CAD build for the part. Positions are in the model's coordinates, mm. A direction names the side the tool comes from. Round coordinates to 2 decimals unless told otherwise and drop trailing zeros. Loops run counter-clockwise (first coordinate to the right, second up) from the corner with the lowest first, then second, coordinate; pieces in that order, holes last.
from build123d import *

# Parameters (mm, degrees)
F1_DEPTH    = 3.175
F2_T1_DEPTH = 41.9033921872
F3_T1_DEPTH = 42.5180012054
F4_T1_DEPTH = 41.9033921872
F5_T1_DEPTH = 41.9033921872


# Not quite as in the source:
# - a fillet or chamfer that OpenCascade refuses, or shapes differently, is made with other operations: its cross-section is extruded or revolved along the edge and cut away or added
# - ends of sketch curves that miss each other by under 0.0002 mm in the source are joined


with BuildPart() as f1:
    # F0 (on Front) → F1 (new body)
    with BuildSketch(Plane.XZ):
        Polygon((-134.9552678654, 118.4551059571), (-242.3083075974, 118.4551059571), (-264.8317917845, 79.4432945156), (-264.8317917845, 5.0669305831), (-242.3083075974, -33.9448883924), (-264.8317917845, -72.9567073679), (-264.8317917845, -147.3330713004), (-242.3083075974, -186.3448902759), (-264.8317917845, -225.3567092514), (-264.8317917845, -299.7330731839), (-242.3083075974, -338.7448921594), (-264.8317917845, -377.7567111349), (-264.8317917845, -452.1330750674), (-242.3083075974, -491.1448940429), (-134.9552678654, -491.1448940429), (-98.2935257718, -427.6448940429), (-24.9700415847, -427.6448940429), (11.6917005088, -491.1448940429), (119.0447402409, -491.1448940429), (155.7064823344, -427.6448940429), (192.3682082155, -427.6448940429), (192.3682082155, -402.2448921594), (155.7064823344, -402.2448921594), (119.0447402409, -338.7448921594), (155.7064823344, -275.2448921594), (192.3682082155, -275.2448921594), (192.3682082155, -249.8448902759), (155.7064823344, -249.8448902759), (119.0447402409, -186.3448902759), (155.7064823344, -122.8448902759), (192.3682082155, -122.8448902759), (192.3682082155, -97.4448883924), (155.7064823344, -97.4448883924), (119.0447402409, -33.9448883924), (155.7064823344, 29.5551116076), (192.3682082155, 29.5551116076), (192.3682082155, 54.9551134911), (155.7064823344, 54.9551134911), (119.0447402409, 118.4551134911), (11.6917005088, 118.4551059571), (-24.9700415847, 54.9551134911), (-98.2935257718, 54.9551134911), align=None)
        Polygon((-261.9552759716, -414.9448940429), (-225.2935338781, -351.4448940429), (-151.970049691, -351.4448940429), (-115.3083075974, -414.9448940429), (-151.970049691, -478.4448940429), (-225.2935338781, -478.4448940429), align=None, mode=Mode.SUBTRACT)
        Polygon((11.6917005088, -338.7448921594), (-24.9700415847, -402.2448921594), (-98.2935257718, -402.2448921594), (-134.9552678654, -338.7448921594), (-98.2935257718, -275.2448921594), (-24.9700415847, -275.2448921594), align=None, mode=Mode.SUBTRACT)
        Polygon((-115.3083075974, -262.5448921594), (-151.970049691, -326.0448921594), (-225.2935338781, -326.0448921594), (-261.9552759716, -262.5448921594), (-225.2935338781, -199.0448921594), (-151.970049691, -199.0448921594), align=None, mode=Mode.SUBTRACT)
        Polygon((138.6917005088, -414.9448940429), (102.0299584153, -478.4448940429), (28.7064742282, -478.4448940429), (-7.9552678654, -414.9448940429), (28.7064742282, -351.4448940429), (102.0299584153, -351.4448940429), align=None, mode=Mode.SUBTRACT)
        Polygon((138.6917005088, -262.5448921594), (102.0299584153, -326.0448921594), (28.7064742282, -326.0448921594), (-7.9552678654, -262.5448921594), (28.7064742282, -199.0448921594), (102.0299584153, -199.0448921594), align=None, mode=Mode.SUBTRACT)
        Polygon((-115.3083075974, -110.1448902759), (-151.970049691, -173.6448902759), (-225.2935338781, -173.6448902759), (-261.9552759716, -110.1448902759), (-225.2935338781, -46.6448902759), (-151.970049691, -46.6448902759), align=None, mode=Mode.SUBTRACT)
        Polygon((11.6917005088, -186.3448902759), (-24.9700415847, -249.8448902759), (-98.2935257718, -249.8448902759), (-134.9552678654, -186.3448902759), (-98.2935257718, -122.8448902759), (-24.9700415847, -122.8448902759), align=None, mode=Mode.SUBTRACT)
        Polygon((11.6917005088, -33.9448883924), (-24.9700415847, -97.4448883924), (-98.2935257718, -97.4448883924), (-134.9552678654, -33.9448883924), (-98.2935257718, 29.5551116076), (-24.9700415847, 29.5551116076), align=None, mode=Mode.SUBTRACT)
        Polygon((-115.3083075974, 42.2551116076), (-151.970049691, -21.2448883924), (-225.2935338781, -21.2448883924), (-261.9552759716, 42.2551116076), (-225.2935338781, 105.7551116076), (-151.970049691, 105.7551116076), align=None, mode=Mode.SUBTRACT)
        Polygon((138.6917005088, -110.1448902759), (102.0299584153, -173.6448902759), (28.7064742282, -173.6448902759), (-7.9552678654, -110.1448902759), (28.7064742282, -46.6448902759), (102.0299584153, -46.6448902759), align=None, mode=Mode.SUBTRACT)
        Polygon((138.6917005088, 42.2551116076), (102.0299584153, -21.2448883924), (28.7064742282, -21.2448883924), (-7.9552678654, 42.2551116076), (28.7064742282, 105.7551116076), (102.0299584153, 105.7551116076), align=None, mode=Mode.SUBTRACT)
    extrude(amount=F1_DEPTH)

    # F2: chamfer of 1.8415 x 3.1895715621 on 1 edges, made by hand

    # F2_s2 → F2_t1 (cut)
    with BuildSketch(Plane.XY.offset(21.3034164558)):
        Polygon((192.3682082155, -3.1895715621), (190.5267082155, 0), (192.3682082155, 0), align=None)
    extrude(amount=F2_T1_DEPTH, mode=Mode.SUBTRACT)

    # F3: chamfer of 1.91008 x 3.3083556065 on 1 edges, made by hand

    # F3_s2 → F3_t1 (cut)
    with BuildSketch(Plane.XY.offset(-131.4038899368)):
        Polygon((190.4581282155, 0), (192.3682082155, -3.3083556065), (192.3682082155, 0), align=None)
    extrude(amount=F3_T1_DEPTH, mode=Mode.SUBTRACT)

    # F4: chamfer of 1.8415 x 3.1895715621 on 1 edges, made by hand

    # F4_s2 → F4_t1 (cut)
    with BuildSketch(Plane.XY.offset(-283.4965873112)):
        Polygon((190.5267082155, 0), (192.3682082155, -3.1895715621), (192.3682082155, 0), align=None)
    extrude(amount=F4_T1_DEPTH, mode=Mode.SUBTRACT)

    # F5: chamfer of 1.8415 x 3.1895715621 on 1 edges, made by hand

    # F5_s2 → F5_t1 (cut)
    with BuildSketch(Plane.XY.offset(-435.8965891948)):
        Polygon((190.5267082155, 0), (192.3682082155, -3.1895715621), (192.3682082155, 0), align=None)
    extrude(amount=F5_T1_DEPTH, mode=Mode.SUBTRACT)


solid = f1.part
Item 1: Mould opens along X. For faces 1 (the flat face through (-253.728, -1.565, -14.166)), 2 (the flat face through (137.12, -1.57, -459.84)), 3 (the flat face through (120.617, -1.565, 10.95)) say: released by +X, released by -X, zero draft, split by the parting line, or undercut.
Verdict:
face 1: released by -X
face 2: released by +X
face 3: undercut
Item 2: Wall check: L1, parallel to Z at x = -37.5, y = -1.55; L2, parallel to Z at x = -163, y = -1.45; L3, parallel to X at y = -2.25, z = -119.5. Give the ranges that are in metal, low to high.
Verdict:
L1: z = -427.64 to -402.24, -275.24 to -249.84, -122.84 to -97.44, 29.56 to 54.96
L2: z = -491.14 to -478.44, -351.44 to -326.04, -199.04 to -173.64, -46.64 to -21.24, 105.76 to 118.46
L3: x = -264.83 to -256.55, -120.71 to -2.55, 133.29 to 191.76
Item 3: Cut at D-D (x = -176). List the corners of the cut face in (y, z) (3 decimals).
Verdict:
outline: (-3.175, -491.145) - (0, -491.145) - (0, -478.445) - (-3.175, -478.445) - close; (-3.175, -351.445) - (0, -351.445) - (0, -326.045) - (-3.175, -326.045) - close; (-3.175, -199.045) - (0, -199.045) - (0, -173.645) - (-3.175, -173.645) - close; (-3.175, -46.645) - (0, -46.645) - (0, -21.245) - (-3.175, -21.245) - close; (-3.175, 105.755) - (0, 105.755) - (0, 118.455) - (-3.175, 118.455) - close
Item 4: Flat gauge pins, fed straight in: P1, Ø1, axis at x = -79.5, y = -1, coming from the +Z side; P2, Ø1.6, axis at x = -78, y = -1, coming from the -Z side. Where does each tip first touch, or does it go through?
Verdict:
P1: stops at z = 54.96
P2: stops at z = -427.64
Item 5: Cut at B-B (z = -281.5). List the corners of the cut face in (x, y) (3 decimals), plus the area to 3 significant figures.
Verdict:
outline: (-264.832, -3.175) - (-251.012, -3.175) - (-251.012, 0) - (-264.832, 0) - close; (-126.252, -3.175) - (-101.905, -3.175) - (-101.905, 0) - (-126.252, 0) - close; (-21.359, -3.175) - (2.988, -3.175) - (2.988, 0) - (-21.359, 0) - close; (127.748, -3.175) - (152.095, -3.175) - (152.095, 0) - (127.748, 0) - close
area: 276 mm2
Item 6: Cut at C-C (x = 129.5). State how many separate pieces and enclosed holes the cut face has, plus the area to 3 significant figures.
Verdict:
separate pieces: 8
enclosed holes: 0
area: 1,070 mm2
Item 7: 3-axis set-ups, long thin cutter, end or side, ignore diameter. For faces 4 (the flat face through (-6.383, -1.565, 87.15)), 5 (the flat face through (137.12, -1.57, -2.64)), 6 (the flat face through (10.632, -1.565, 10.061)): which of +Z, -Z, +X, -X, +Y, -Y reach the whole face in a straight line?
Verdict:
face 4: +Z, +Y, -Y
face 5: +X, +Y, -Y
face 6: +Y, -Y
Item 8: Cut at A-A (x = -66.5). List the corners of the cut face in (y, z) (3 decimals), plus the area to 3 significant figures.
Verdict:
outline: (-3.175, -427.645) - (0, -427.645) - (0, -402.245) - (-3.175, -402.245) - close; (-3.175, -275.245) - (0, -275.245) - (0, -249.845) - (-3.175, -249.845) - close; (-3.175, -122.845) - (0, -122.845) - (0, -97.445) - (-3.175, -97.445) - close; (-3.175, 29.555) - (0, 29.555) - (0, 54.955) - (-3.175, 54.955) - close
area: 323 mm2
